Here's the drawing with two shaded views (mm, measured from the low corner). I have some questions. Coordinates: 2 decimals unless noted, no trailing zeros. Write each loop counter-clockwise with the first axis right and the second up, starting at its lowest first coordinate (ties: lowest second). Pieces come first, ordered by that corner, then holes. Notation, with made-up numbers: (78, 26.25) - (117, 26.25) arc R17 cw to (117, 41.25) - close; hole circle Ø4 at (41.5, -1.75). An arc over 180 degrees is marked (long way). Answer in a Markdown table with one row per item. Add a question column.
Item 1: I'm going to push flat-ended pins straight in: pin 1 (1.5 mm diameter, centred on y = 26, z = 1, fed in from -X); pin 2 (1.5 mm diameter, centred on x = 31, z = 1.5, fed in from +Y); pin 3 (1.5 mm diameter, centred on x = 30.5, z = 1.5, fed in from -Y). Where does each tip first touch, or does it pass through?
Item 2: If I drill on probe 1 along Y at (x, z) = (27.25, 1.9) (3 decimals); probe 2 along Y at (x, z) = (28.5, 0.2); probe 3 along X at (y, z) = (12, 2.6), over which ranges is the centre line in solid material (lowest first)? Write a range as from..to.
Item 3: Imagine slicing it at C-C (z = 1.05). Please give me the cut outline in (x, y) (3 decimals), plus the area to 3 significant figures.
Item 4: Imagine slicing it at A-A (y = 27.25). Please give me the cut outline in (x, z).
Item 5: Imagine slicing it at B-B (x = 27.25). Please give me the cut outline in (y, z) (3 decimals).
Item 6: Imagine slicing it at D-D (x = 11). Please give me the cut outline in (y, z).
Item 7: We'd pull the mould along X, two halves only. Please class the marked faces 1 and 2: +X half, -X half, draft (parallel to the pull), parting line (faces both ways), or undercut.
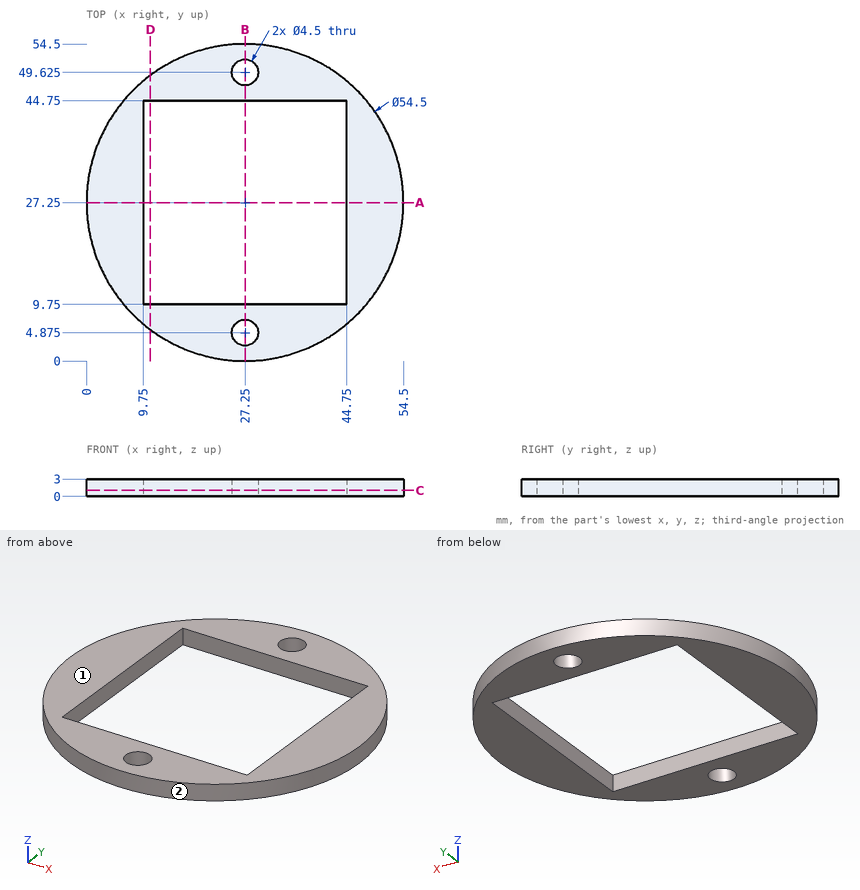
Here are the results:
| question | item | result |
|---|---|---|
| 1 | pin 1 | stops at x = 0 |
| 1 | pin 2 | stops at y = 54.33 |
| 1 | pin 3 | stops at y = 0.11 |
| 2 | probe 1 | y = 0..2.625, 7.125..9.75, 44.75..47.375, 51.875..54.5 |
| 2 | probe 2 | y = 0.03..3, 6.75..9.75, 44.75..47.75, 51.5..54.47 |
| 2 | probe 3 | x = 4.67..9.75, 44.75..49.83 |
| 3 | outline | circle Ø54.5 at (27.25, 27.25); hole (9.75, 9.75) - (44.75, 9.75) - (44.75, 44.75) - (9.75, 44.75) - close; hole circle Ø4.5 at (27.25, 4.875); hole circle Ø4.5 at (27.25, 49.625) |
| 3 | area | 1,080 mm2 |
| 4 | outline | (0, 0) - (9.75, 0) - (9.75, 3) - (0, 3) - close; (44.75, 0) - (54.5, 0) - (54.5, 3) - (44.75, 3) - close |
| 5 | outline | (0, 0) - (2.625, 0) - (2.625, 3) - (0, 3) - close; (7.125, 0) - (9.75, 0) - (9.75, 3) - (7.125, 3) - close; (44.75, 0) - (47.375, 0) - (47.375, 3) - (44.75, 3) - close; (51.875, 0) - (54.5, 0) - (54.5, 3) - (51.875, 3) - close |
| 6 | outline | (5.38, 0) - (9.75, 0) - (9.75, 3) - (5.38, 3) - close; (44.75, 0) - (49.12, 0) - (49.12, 3) - (44.75, 3) - close |
| 7 | face 1 | draft |
| 7 | face 2 | parting line |
